The model under review builds one solid part; all positions refer to its coordinate system, in mm. A direction names the side the tool comes from. Give positions to 0.01 mm unless a question says otherwise; leave off trailing zeros. Write each loop counter-clockwise with the first axis right and the second up, starting at its lowest first coordinate (ties: lowest second). Pieces come first, ordered by that corner, then holes. Notation, with made-up numbers: (89, 18.25) - (124, 18.25) arc R10 cw to (124, 26.25) - close; hole circle Ø7 at (13.25, 56). An arc over 180 degrees is marked (long way). Write item = value, one per line.
```python
from build123d import *

# Parameters (mm, degrees)
F0_R     = 30
F0_R_2   = 3.3
F1_DEPTH = 8
F2_R     = 6
F3_DEPTH = 4
F4_R     = 12.5
F5_DEPTH = 5
F6_R     = 3.15
F7_DEPTH = 8
F9_DEPTH = 25.4


with BuildPart() as f1:
    # F0 (on Front) → F1 (new body)
    with BuildSketch(Plane.XZ):
        Circle(F0_R)
        with Locations((0, -20)):
            Circle(F0_R_2, mode=Mode.SUBTRACT)
        with Locations((-20, 0)):
            Circle(F0_R_2, mode=Mode.SUBTRACT)
        with Locations((20, 0)):
            Circle(F0_R_2, mode=Mode.SUBTRACT)
        with Locations((0, 20)):
            Circle(F0_R_2, mode=Mode.SUBTRACT)
    extrude(amount=F1_DEPTH)

    # F2 (on face) → F3 (cut)
    with BuildSketch(Plane.XZ.offset(8)):
        with Locations((0, 20)):
            Circle(F2_R)
        with Locations((-20, 0)):
            Circle(F2_R)
        with Locations((20, 0)):
            Circle(F2_R)
        with Locations((0, -20)):
            Circle(F2_R)
    extrude(amount=-F3_DEPTH, mode=Mode.SUBTRACT)

    # F4 (on face) → F5 (join)
    with BuildSketch(Plane.XZ.offset(8)):
        Circle(F4_R)
    extrude(amount=F5_DEPTH)

    # F6 (on face) → F7 (join)
    with BuildSketch(Plane.XZ.offset(13)):
        Circle(F6_R)
    extrude(amount=F7_DEPTH)

    # F8 (on face) → F9 (cut)
    with BuildSketch(Plane.XZ.offset(8)):
        with BuildLine():
            ThreePointArc((-13.324728, 8.62944), (-11.22532, 11.22532), (-8.62944, 13.324728))
            ThreePointArc((-8.62944, 13.324728), (-7.568985, 14.755035), (-7.708129, 16.530135))
            Line((-7.708129, 16.530135), (-9.601232, 20.589909))
            ThreePointArc((-9.601232, 20.589909), (-11.168675, 21.947918), (-13.225838, 21.684954))
            ThreePointArc((-13.225838, 21.684954), (-17.960512, 17.960512), (-21.684954, 13.225838))
            ThreePointArc((-21.684954, 13.225838), (-21.947918, 11.168675), (-20.589909, 9.601232))
            Line((-20.589909, 9.601232), (-16.530135, 7.708129))
            ThreePointArc((-16.530135, 7.708129), (-14.755035, 7.568985), (-13.324728, 8.62944))
        make_face()
        with BuildLine():
            ThreePointArc((-20.589909, -9.601232), (-21.947918, -11.168675), (-21.684954, -13.225838))
            ThreePointArc((-21.684954, -13.225838), (-17.960512, -17.960512), (-13.225838, -21.684954))
            ThreePointArc((-13.225838, -21.684954), (-11.168675, -21.947918), (-9.601232, -20.589909))
            Line((-9.601232, -20.589909), (-7.708129, -16.530135))
            ThreePointArc((-7.708129, -16.530135), (-7.568985, -14.755035), (-8.62944, -13.324728))
            ThreePointArc((-8.62944, -13.324728), (-11.22532, -11.22532), (-13.324728, -8.62944))
            ThreePointArc((-13.324728, -8.62944), (-14.755035, -7.568985), (-16.530135, -7.708129))
            Line((-16.530135, -7.708129), (-20.589909, -9.601232))
        make_face()
        with BuildLine():
            ThreePointArc((9.601232, -20.589909), (11.168675, -21.947918), (13.225838, -21.684954))
            ThreePointArc((13.225838, -21.684954), (17.960512, -17.960512), (21.684954, -13.225838))
            ThreePointArc((21.684954, -13.225838), (21.947918, -11.168675), (20.589909, -9.601232))
            Line((20.589909, -9.601232), (16.530135, -7.708129))
            ThreePointArc((16.530135, -7.708129), (14.755035, -7.568985), (13.324728, -8.62944))
            ThreePointArc((13.324728, -8.62944), (11.22532, -11.22532), (8.62944, -13.324728))
            ThreePointArc((8.62944, -13.324728), (7.568985, -14.755035), (7.708129, -16.530135))
            Line((7.708129, -16.530135), (9.601232, -20.589909))
        make_face()
        with BuildLine():
            ThreePointArc((20.589909, 9.601232), (21.947918, 11.168675), (21.684954, 13.225838))
            ThreePointArc((21.684954, 13.225838), (17.960512, 17.960512), (13.225838, 21.684954))
            ThreePointArc((13.225838, 21.684954), (11.168675, 21.947918), (9.601232, 20.589909))
            Line((9.601232, 20.589909), (7.708129, 16.530135))
            ThreePointArc((7.708129, 16.530135), (7.568985, 14.755035), (8.62944, 13.324728))
            ThreePointArc((8.62944, 13.324728), (11.22532, 11.22532), (13.324728, 8.62944))
            ThreePointArc((13.324728, 8.62944), (14.755035, 7.568985), (16.530135, 7.708129))
            Line((16.530135, 7.708129), (20.589909, 9.601232))
        make_face()
    extrude(amount=-F9_DEPTH, mode=Mode.SUBTRACT)


solid = f1.part
```
1. Machinability: for faces 1 (the cylindrical face through (11.26, -4.06, -11.19)), 2 (the cylindrical face through (-0.78, -6.03, -14.05)), which of the approach directions +Z, -Z, +X, -X, +Y, -Y give a long, thin tool a straight path to every point of the face, cutting with its end or side? Answer none if there is none.
Findings below:
face_1 = +Y, -Y
face_2 = -Y
2. Take a section at B-B on x = 0. Give the boundary of the cut face in (y, z).
Findings below:
outline = (-21, -3.15) - (-13, -3.15) - (-13, -12.5) - (-8, -12.5) - (-8, -14) - (-4, -14) - (-4, -16.7) - (0, -16.7) - (0, 16.7) - (-4, 16.7) - (-4, 14) - (-8, 14) - (-8, 12.5) - (-13, 12.5) - (-13, 3.15) - (-21, 3.15) - close; (-8, -30) - (0, -30) - (0, -23.3) - (-4, -23.3) - (-4, -26) - (-8, -26) - close; (-8, 26) - (-4, 26) - (-4, 23.3) - (0, 23.3) - (0, 30) - (-8, 30) - close
3. Insertion check: P1, Ø5, axis at x = 21, y = -5, coming from the +Z side; P2, Ø9.5, axis at x = -2.5, z = -20, coming from the -Y side; P3, Ø8, axis at y = -12.5, z = -3, coming from the -X side; P4, Ø5.5, axis at x = 20, z = 0, coming from the +Y side. Each pin has a flat end and moves straight along its axis. Give the tip position at first contact, or say it passes through.
Findings below:
P1 = 23.62
P2 = -8
P3 = -12.5
P4 = through
4. Draft analysis for pull direction X (two halves, no side actions). For faces 3 (the cylindrical face through (-18.02, -4.06, -17.9)), 4 (the flat face through (0, -21, 0)), 5 (the cylindrical face through (-2.5, -16.944, -1.917)), state which applies: +X half, -X half, draft (parallel to the pull), parting line (faces both ways), or undercut.
Findings below:
face_3 = undercut
face_4 = draft
face_5 = parting line
5. Take a section at C-C on y = -2.25. Count the separate pieces of the cut face and the enclosed holes in it, and give its area (3 significant figures).
Findings below:
separate_pieces = 1
enclosed_holes = 8
area = 2,160 mm²
6. For line 1 (Z direction, x = 0, y = -6.6); line 2 (Z direction, x = 0, y = -3.2); line 3 (X direction, y = -7.5, z = -5.5), list the stretches that pass through material, from the lowest coordinate up. Write a range as from..to.
Findings below:
line_1 = -30..-26, -14..14, 26..30
line_2 = -30..-23.3, -16.7..16.7, 23.3..30
line_3 = -29.49..-22.4, -17.6..17.6, 22.4..29.49
7. Take a section at D-D on z = -11. Give the boundary of the cut face in (x, y).
Findings below:
outline = (-27.91, -8) - (-21.89, -8) - (-21.89, 0) - (-27.91, 0) - close; (-11.45, -8) - (-5.94, -8) - (-5.94, -13) - (5.94, -13) - (5.94, -8) - (11.45, -8) - (11.45, 0) - (-11.45, 0) - close; (21.89, -8) - (27.91, -8) - (27.91, 0) - (21.89, 0) - close
8. Take a section at A-A on z = 0. Give the boundary of the cut face in (x, y).
Findings below:
outline = (-30, -8) - (-26, -8) - (-26, -4) - (-23.3, -4) - (-23.3, 0) - (-30, 0) - close; (-16.7, -4) - (-14, -4) - (-14, -8) - (-12.5, -8) - (-12.5, -13) - (-3.15, -13) - (-3.15, -21) - (3.15, -21) - (3.15, -13) - (12.5, -13) - (12.5, -8) - (14, -8) - (14, -4) - (16.7, -4) - (16.7, 0) - (-16.7, 0) - close; (23.3, -4) - (26, -4) - (26, -8) - (30, -8) - (30, 0) - (23.3, 0) - close
